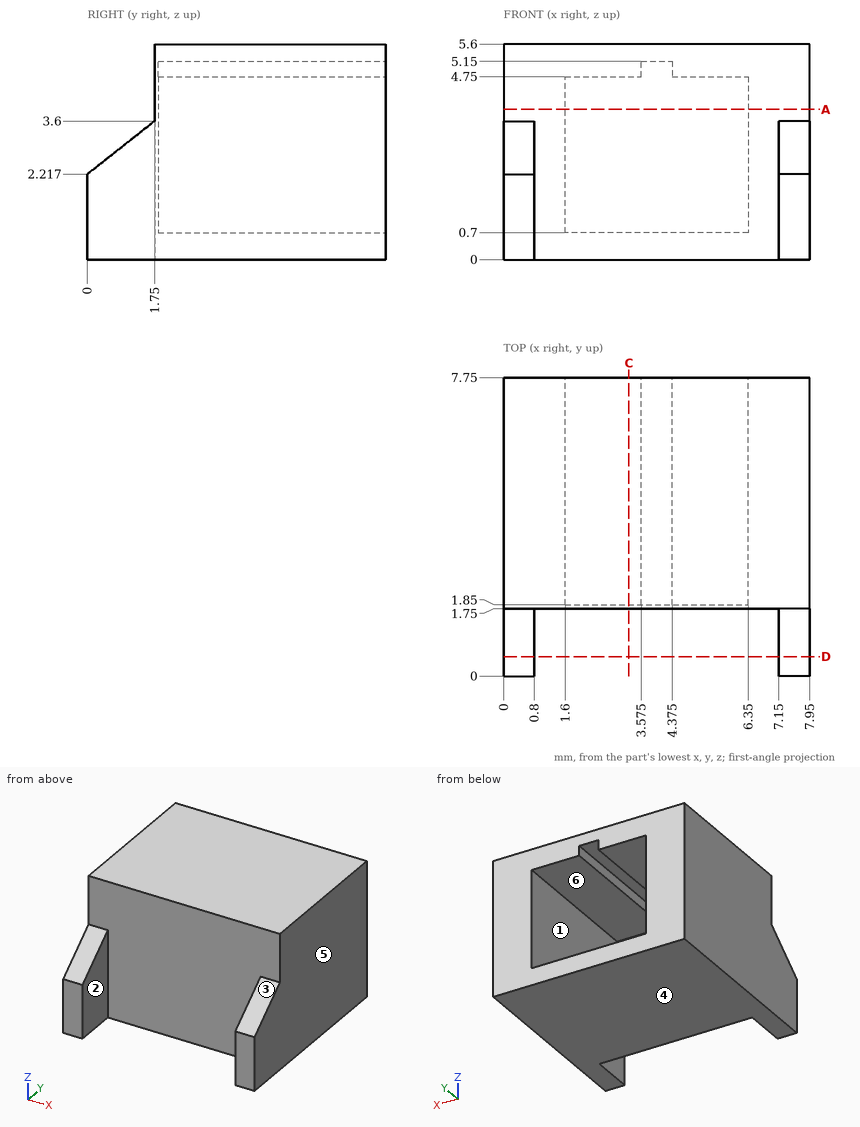
Source: three-view drawing plus pictorial views. Frame: mm from the lowest corner of the part. A direction names the side the tool comes from. Round coordinates to 2 decimals unless told otherwise and drop trailing zeros. Loops run counter-clockwise (first coordinate to the right, second up) from the corner with the lowest first, then second, coordinate; pieces in that order, holes last. Notation, with made-up numbers: (8.5, -28.75) - (41.5, -28.75) arc R8 ccw to (41.5, -13.75) - close; hole circle Ø2 at (-24.75, 27.5). An arc over 180 degrees is marked (long way). Write each question's results on one line, items separated by ' | '. Start each with the question number.
1) Access query for the marked faces 1, 2 and 3. Directions: +Z, -Z, +X, -X, +Y, -Y. A direction counts if a zero-diameter tool reaches every point of the face in a straight line with its end or side. Return the directions, or none.
2) Mould query, pull axis Z, two halves, no side actions, for the marked faces 4, 5 and 6. Classes: released by +Z, released by -Z, zero draft, split by the parting line, or undercut.
3) Cut plane C-C on x = 3.25. Return loops of the section in (y, z).
4) Cut plane D-D on y = 0.5. Return loops of the section in (x, z).
5) First-contact query: P1, Ø1.7, axis at x = 2.5, z = 2.5, coming from the -Y side; P2, Ø2, axis at x = 4, z = 2, coming from the +Y side. Flat tips, straight axial feed; report the tip coordinate or a pass-through.
6) Cut plane A-A on z = 3.9. Return loops of the section in (x, y).
7) Line query: probe 1 along X at (y, z) = (4, 0.75); probe 2 along Z at (x, y) = (4, 6.75); probe 3 along X at (y, z) = (1, 2.55). Output: solid intervals per line, ascending. Write a range as [from, to].
Verdict:
1) face 1: +Y | face 2: +Z, -Z, -Y | face 3: +Z, +X, -X, -Y
2) face 4: released by -Z | face 5: zero draft | face 6: undercut
3) outline: (1.75, 0) - (7.75, 0) - (7.75, 0.7) - (1.85, 0.7) - (1.85, 4.75) - (7.75, 4.75) - (7.75, 5.6) - (1.75, 5.6) - close
4) outline: (0, 0) - (0.8, 0) - (0.8, 2.61) - (0, 2.61) - close; (7.15, 0) - (7.95, 0) - (7.95, 2.61) - (7.15, 2.61) - close
5) P1: stops at y = 1.75 | P2: stops at y = 1.85
6) outline: (0, 1.75) - (7.95, 1.75) - (7.95, 7.75) - (6.35, 7.75) - (6.35, 1.85) - (1.6, 1.85) - (1.6, 7.75) - (0, 7.75) - close
7) probe 1: x = [0, 1.6], [6.35, 7.95] | probe 2: z = [0, 0.7], [5.15, 5.6] | probe 3: x = [0, 0.8], [7.15, 7.95]
